Autodesk Inventor part; units mm, degrees
ref_plane "Work Plane1" through (0, 0, 10) normal (0, 0, 1) x (1, 0, 0)
ref_plane "YZ Plane" through (0, 0, 0) normal (1, 0, 0) x (0, 1, 0)
ref_plane "XZ Plane" through (0, 0, 0) normal (0, 1, 0) x (-1, 0, 0)
ref_plane "Work Plane1" through (0, 0, 10) normal (0, 0, 1) x (1, 0, 0)
sketch "Sketch1" plane through (0, 0, 10) normal (0, 0, 1) x (1, 0, 0)
  line L0 (-4.0299, -0.3538) -> (-2.2322, 1.4439) construction
  arc A0 (-1.4439, 2.2322) -> (-2.2322, 1.4439) centre (-0.9299, 0.9299) ccw construction
  line L1 (-1.4439, 2.2322) -> (0.3538, 4.0299) construction
  line L2 (-37.8299, 42.8299) -> (-37.8299, 37.8299) construction
  line L3 (-37.8299, 37.8299) -> (-42.9208, 37.8299) construction
  line L4 (-37.8299, 42.2137) -> (-37.8299, 45.8299) construction
  line L5 (-37.8299, 45.8299) -> (-4.0299, 45.8299) construction
  line L6 (-4.0299, 45.8299) -> (-4.0299, 42.2137) construction
  line L7 (-4.0299, 4.0299) -> (0.3538, 4.0299)
  circle A1 centre (-20.9299, 20.9299) radius 17.5
  line L8 (-20.9299, 58.9723) -> (17.1124, 20.9299) construction
  line L9 (17.1124, 20.9299) -> (-20.9299, -17.1124) construction
  line L10 (-20.9299, -17.1124) -> (-58.9723, 20.9299) construction
  line L11 (-58.9723, 20.9299) -> (-20.9299, 58.9723) construction
  line L12 (-20.9299, 58.9723) -> (-20.9299, -17.1124) construction
  line L13 (17.1124, 20.9299) -> (-58.9723, 20.9299) construction
  line L14 (-20.9299, 58.9723) -> (32.8701, 58.9723) construction
  line L15 (-43.4299, 43.4299) -> (1.5701, 43.4299) construction
  line L16 (1.5701, 43.4299) -> (1.5701, -1.5701) construction
  line L17 (1.5701, -1.5701) -> (-43.4299, -1.5701) construction
  line L18 (-43.4299, -1.5701) -> (-43.4299, 43.4299) construction
  line L19 (-43.4299, 43.4299) -> (1.5701, -1.5701) construction
  line L20 (1.5701, 43.4299) -> (-43.4299, -1.5701) construction
  line L21 (-43.4299, 5.3876) -> (-43.4299, 36.4723)
  line L22 (-43.4299, 36.4723) -> (-36.4723, 43.4299)
  line L23 (-36.4723, 43.4299) -> (-5.3876, 43.4299)
  line L24 (-5.3876, 43.4299) -> (1.5701, 36.4723)
  line L25 (1.5701, 36.4723) -> (1.5701, 5.3876)
  line L26 (1.5701, 5.3876) -> (-5.3876, -1.5701)
  line L27 (-5.3876, -1.5701) -> (-36.4723, -1.5701)
  line L28 (-36.4723, -1.5701) -> (-43.4299, 5.3876)
  line L29 (-4.0299, 42.2137) -> (-37.8299, 42.2137)
  line L30 (-4.0299, -0.3538) -> (-4.0299, 4.0299)
  circle A2 centre (-20.9299, 20.9299) radius 1.5
  line L31 (-10.9299, 10.9299) -> (-30.9299, 10.9299) construction
  line L32 (-30.9299, 10.9299) -> (-30.9299, 30.9299) construction
  line L33 (-30.9299, 30.9299) -> (-10.9299, 30.9299) construction
  line L34 (-10.9299, 30.9299) -> (-10.9299, 10.9299) construction
  line L35 (-10.9299, 10.9299) -> (-30.9299, 30.9299) construction
  line L36 (-30.9299, 10.9299) -> (-10.9299, 30.9299) construction
  circle A3 centre (-30.9299, 30.9299) radius 1.4
  circle A4 centre (-30.9299, 10.9299) radius 1.4
  circle A5 centre (-10.9299, 10.9299) radius 1.4
  line L37 (-45.8299, 37.8299) -> (-42.0723, 37.8299) construction
  line L38 (-42.1723, 37.7299) -> (-45.8299, 37.7299)
  line L39 (-45.8299, 37.7299) -> (-45.8299, 4.1299)
  line L40 (-45.8299, 4.1299) -> (-42.1723, 4.1299)
  line L41 (-42.1723, 4.1299) -> (-42.1723, 37.7299)
  line L42 (-45.8299, 4.0299) -> (-42.0723, 4.0299) construction
  line L43 (-45.8299, 37.8299) -> (-42.0723, 37.8299)
  line L44 (-37.7299, 45.8299) -> (-4.1299, 45.8299)
  line L45 (-4.1299, 45.8299) -> (-4.1299, 42.1723)
  line L46 (-4.1299, 42.1723) -> (-37.7299, 42.1723)
  line L47 (-37.7299, 42.1723) -> (-37.7299, 45.8299)
  line L48 (0.4701, 37.8299) -> (0.4701, 4.0299) construction
  line L49 (0.4701, 4.0299) -> (3.9701, 4.0299) construction
  line L50 (3.9701, 37.8299) -> (3.9701, 4.0299) construction
  line L51 (0.4701, 37.8299) -> (3.9701, 37.8299) construction
  line L52 (-45.8299, -3.9701) -> (-4.0299, -3.9701) construction
  line L53 (0.3124, 37.7299) -> (3.9701, 37.7299)
  line L54 (3.9701, 37.7299) -> (3.9701, 4.1299)
  line L55 (3.9701, 4.1299) -> (0.3124, 4.1299)
  line L56 (0.3124, 4.1299) -> (0.3124, 37.7299)
  line L57 (-4.1713, -0.3538) -> (-37.7299, -0.3538)
  line L58 (-37.7299, -0.3538) -> (-37.7299, -3.9701)
  line L59 (-37.7299, -3.9701) -> (-4.1713, -3.9701)
  line L60 (-4.1713, -3.9701) -> (-4.1713, -0.3538)
  point P0 (-37.8299, 4.0299)
  dimension "d18" = 53.8
  dimension "d19" = 45
  dimension "d20" = 53.8
  dimension "d21" = 45
  dimension "d22" = 45
  dimension "d30" = 20
  dimension "d31" = 20
  dimension "d32" = 2.8
  dimension "d33" = 2.8
  dimension "d34" = 2.8
  dimension "d35" = 3
  dimension "d36" = 0.1
  dimension "d37" = 0.1
  dimension "d38" = 0.1
  dimension "d39" = 0.1
extrude "Extrusion1" add sketch "Sketch1" along normal blind 11 contours L30 L26 L57 L28 L41 L22 L46 L24 L56 L7 | L7 L26 L30 | L56 L24 L25 L26 | L26 L25 L24 L53 L54 L55 | L60 L59 L58 L57 L28 L27 L26 | L26 L27 L28 L57 | L46 L22 L29 L24 | L24 L29 L45 | L40 L39 L38 L22 L21 L28 | L28 L21 L22 L41 | L29 L22 L23 L24 | L24 L23 L22 L29 L47 L44 L45 | L47 L29 L22 | A1 | A2 | A3 | A4 | A5
sketch "Skizze4" plane through (0, 0, 21) normal (0, 0, 1) x (1, 0, 0)
  line L0 (-37.7299, 42.1723) -> (-42.1723, 37.7299)
  line L1 (-42.1723, 37.7299) -> (-45.8299, 37.7299)
  line L2 (-45.8299, 37.7299) -> (-45.8299, 4.1299) construction
  line L3 (-45.8299, 4.1299) -> (-42.1723, 4.1299)
  line L4 (-42.1723, 4.1299) -> (-37.6885, -0.3538)
  line L5 (-37.6885, -0.3538) -> (-37.7299, -0.3538)
  line L6 (-37.7299, -0.3538) -> (-37.7299, -3.9701)
  line L7 (-37.7299, -3.9701) -> (-4.1713, -3.9701) construction
  line L8 (-4.1713, -3.9701) -> (-4.1713, -0.3538)
  line L9 (-4.1713, -0.3538) -> (0.3124, 4.1299)
  line L10 (0.3124, 4.1299) -> (3.9701, 4.1299)
  line L11 (3.9701, 4.1299) -> (3.9701, 37.7299) construction
  line L12 (3.9701, 37.7299) -> (0.3124, 37.7299)
  line L13 (0.3124, 37.7299) -> (-4.1299, 42.1723)
  line L14 (-4.1299, 42.1723) -> (-4.1299, 45.8299)
  line L15 (-4.1299, 45.8299) -> (-37.7299, 45.8299) construction
  line L16 (-37.7299, 45.8299) -> (-37.7299, 42.1723)
  line L17 (-37.9299, 46.0299) -> (-3.9299, 46.0299) construction
  line L18 (-3.9299, 46.0299) -> (-3.9299, 42.2551)
  line L19 (-3.9299, 42.2551) -> (0.3953, 37.9299)
  line L20 (0.3953, 37.9299) -> (4.1701, 37.9299)
  line L21 (4.1701, 37.9299) -> (4.1701, 3.9299) construction
  line L22 (4.1701, 3.9299) -> (0.3953, 3.9299)
  line L23 (0.3953, 3.9299) -> (-3.9713, -0.4367)
  line L24 (-3.9713, -0.4367) -> (-3.9713, -4.1701)
  line L25 (-3.9713, -4.1701) -> (-37.9299, -4.1701) construction
  line L26 (-37.9299, -4.1701) -> (-37.9299, -0.3953)
  line L27 (-37.9299, -0.3953) -> (-42.2551, 3.9299)
  line L28 (-42.2551, 3.9299) -> (-46.0299, 3.9299)
  line L29 (-46.0299, 3.9299) -> (-46.0299, 37.9299) construction
  line L30 (-46.0299, 37.9299) -> (-42.2551, 37.9299)
  line L31 (-42.2551, 37.9299) -> (-37.9299, 42.2551)
  line L32 (-37.9299, 42.2551) -> (-37.9299, 46.0299)
  line L33 (-45.8299, 37.7299) -> (-45.8299, 37.9299)
  line L34 (-4.1299, 45.8299) -> (-37.7299, 45.8299)
  line L35 (-37.7299, 45.8299) -> (-37.9299, 45.8299)
  line L36 (-4.1299, 45.8299) -> (-3.9299, 45.8299)
  line L37 (3.9701, 37.7299) -> (3.9701, 37.9299)
  line L38 (3.9701, 4.1299) -> (3.9701, 37.7299)
  line L39 (3.9701, 4.1299) -> (3.9701, 3.9299)
  line L40 (-4.1713, -3.9701) -> (-3.9713, -3.9701)
  line L41 (-37.7299, -3.9701) -> (-37.9299, -3.9701)
  line L42 (-45.8299, 4.1299) -> (-45.8299, 3.9299)
  point P0 (0, 0)
  dimension "d40" = 0.2
extrude "IM_offset" add sketch "Skizze4" against normal up to surface (11 mm away)
ref_plane "Arbeitsebene5" through (-20.9299, 3.9299, 10) normal (1, 0, 0) x (0, 0, -1)
ref_plane "Arbeitsebene6" through (-37.9299, 20.9299, 10) normal (0, 1, 0) x (1, 0, 0)
sketch "Skizze25" plane through (0, 0, 21) normal (0, 0, 1) x (1, 0, 0)
  arc A0 (-35.9433, 11.4849) -> (-11.4049, 36.0233) centre (-20.9299, 21.0099) ccw
  circle A1 centre (-20.9299, 21.0099) radius 17.78
  circle A2 centre (-20.9299, 21.0099) radius 13
  point P0 (0, 0)
  point P1 (-11.4049, 36.0233)
  dimension "d152" = 26
extrude "Extrusion21" cut sketch "Skizze25" against normal blind 12 contours A2
sketch "Skizze26" plane through (0, 0, 21) normal (0, 0, 1) x (1, 0, 0)
  line L0 (-43.7899, 28.1537) -> (-43.7899, 13.8662)
  arc A0 (-43.7899, 13.8662) -> (-41.4087, 11.4849) centre (-41.4087, 13.8662) ccw
  line L1 (-41.4087, 11.4849) -> (-35.9433, 11.4849)
  arc A1 (-35.9433, 11.4849) -> (-11.4049, 36.0233) centre (-20.9299, 21.0099) ccw
  line L2 (-11.4049, 36.0233) -> (-11.4049, 41.4887)
  arc A2 (-11.4049, 41.4887) -> (-13.7862, 43.8699) centre (-13.7862, 41.4887) ccw
  line L3 (-13.7862, 43.8699) -> (-28.0737, 43.8699)
  arc A3 (-28.0737, 43.8699) -> (-30.4549, 41.4887) centre (-28.0737, 41.4887) ccw
  line L4 (-30.4549, 41.4887) -> (-30.4549, 36.0233)
  arc A4 (-30.4549, 36.0233) -> (-35.9433, 30.5349) centre (-20.9299, 21.0099) ccw
  line L5 (-35.9433, 30.5349) -> (-41.4087, 30.5349)
  arc A5 (-41.4087, 30.5349) -> (-43.7899, 28.1537) centre (-41.4087, 28.1537) ccw
  circle A6 centre (-20.9299, 21.0099) radius 13.2911
  point P0 (0, 0)
extrude "Extrusion22" cut sketch "Skizze26" against normal blind 9.2 contours A5 L5 A4 L4 A3 L3 A2 L2 A1 L1 A0 L0 | A6
sketch "Skizze27" plane through (-37.9299, -3.9701, 10) normal (0, -1, 0) x (1, 0, 0)
  line L0 (33.9586, 0) -> (0, 0)
  line L1 (33.9586, 11) -> (33.9586, 0)
  line L2 (33.9586, 11) -> (0, 11)
  line L3 (0, 11) -> (0, 0)
  circle A0 centre (16.9793, 6) radius 2.85
  point P0 (37.9299, -10)
  dimension "d155" = 5.7
hole "Bohrung1" at (-20.9506, -3.9701, 16) direction (0, 1, 0) diameter 4.5 depth 30 tip angle 118 counterbore diameter 5.7 counterbore depth 5.8
sketch "Skizze28" plane through (0, 0, 21) normal (0, 0, 1) x (1, 0, 0)
  line L0 (-35.9433, 11.4849) -> (-41.4087, 11.4849)
  arc A0 (-43.7899, 13.8662) -> (-41.4087, 11.4849) centre (-41.4087, 13.8662) ccw
  line L1 (-43.7899, 13.8662) -> (-43.7899, 28.1537)
  arc A1 (-41.4087, 30.5349) -> (-43.7899, 28.1537) centre (-41.4087, 28.1537) ccw
  line L2 (-41.4087, 30.5349) -> (-35.9433, 30.5349)
  arc A2 (-30.4549, 36.0233) -> (-35.9433, 30.5349) centre (-20.9299, 21.0099) ccw
  line L3 (-30.4549, 36.0233) -> (-30.4549, 41.4887)
  arc A3 (-28.0737, 43.8699) -> (-30.4549, 41.4887) centre (-28.0737, 41.4887) ccw
  line L4 (-28.0737, 43.8699) -> (-13.7862, 43.8699)
  arc A4 (-11.4049, 41.4887) -> (-13.7862, 43.8699) centre (-13.7862, 41.4887) ccw
  line L5 (-11.4049, 41.4887) -> (-11.4049, 36.0233)
  arc A5 (-35.9433, 11.4849) -> (-11.4049, 36.0233) centre (-20.9299, 21.0099) ccw
  line L6 (3.9701, 3.9299) -> (3.9701, 37.9299)
  line L7 (3.9701, 37.9299) -> (0.3953, 37.9299)
  line L8 (0.3953, 37.9299) -> (-3.9299, 42.2551)
  line L9 (-3.9299, 42.2551) -> (-3.9299, 45.8299)
  line L10 (-3.9299, 45.8299) -> (-37.9299, 45.8299)
  line L11 (-37.9299, 45.8299) -> (-37.9299, 42.2551)
  line L12 (-37.9299, 42.2551) -> (-42.2551, 37.9299)
  line L13 (-42.2551, 37.9299) -> (-45.8299, 37.9299)
  line L14 (-45.8299, 37.9299) -> (-45.8299, 3.9299)
  line L15 (-42.2551, 3.9299) -> (-45.8299, 3.9299)
  line L16 (-37.9299, -0.3953) -> (-42.2551, 3.9299)
  line L17 (-37.9299, -3.9701) -> (-37.9299, -0.3953)
  line L18 (-3.9713, -3.9701) -> (-37.9299, -3.9701)
  line L19 (-3.9713, -3.9701) -> (-3.9713, -0.4367)
  line L20 (-3.9713, -0.4367) -> (0.3953, 3.9299)
  line L21 (0.3953, 3.9299) -> (3.9701, 3.9299)
  circle A6 centre (-1.2449, 9.5799) radius 2.0828
  circle A7 centre (-1.2449, 32.4399) radius 2.0828
  circle A8 centre (-40.6149, 32.4399) radius 2.0828
  circle A9 centre (-40.6149, 9.5799) radius 2.0828
  point P0 (0, 0)
hole "Bohrung2" at (-40.6149, 9.5799, 21) at (-40.6149, 32.4399, 21) at (-1.2449, 32.4399, 21) at (-1.2449, 9.5799, 21) direction (0, 0, -1) diameter 2.8 depth 30 tip angle 118
sketch "Skizze29" plane through (-28.0737, 43.8699, 21) normal (0, -1, 0) x (1, 0, 0)
  circle A0 centre (7.123, -5) radius 2.85
  circle A1 centre (7.123, -5) radius 4.25
  point P0 (28.0737, -21)
  dimension "d173" = 8.5
extrude "Extrusion23" cut sketch "Skizze29" against normal blind 1 contours A0 | A1
pattern_circular "Runde Anordnung1" count 2 over 90 about axis through (-20.9299, 21.0099, 21) along (0, 0, 1) of "Bohrung1", "Extrusion23"
properties part number "20_Cube_Insert_Filter_25mm"
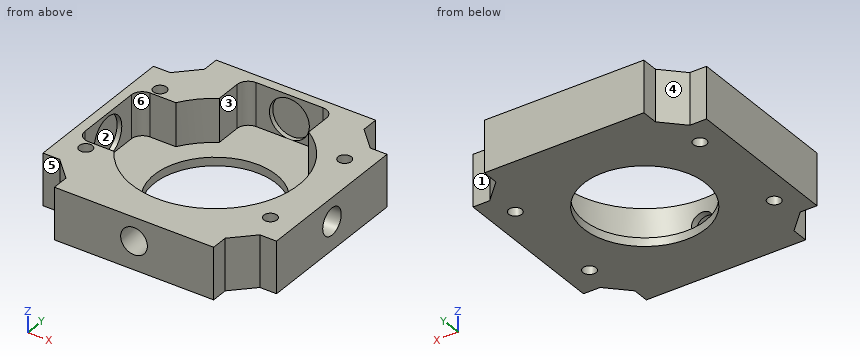
Geometry: final body of the model. Coordinates: model frame, mm. Face numbers are marked on the shaded views. A direction names the side the tool comes from. Round coordinates to 2 decimals unless told otherwise and drop trailing zeros. Order: outer loops, then holes, each group sorted by start corner. A loop starts at its lowest first (then second) coordinate and runs counter-clockwise, first axis right, second up. Notation, with made-up numbers: (-18.5, -10) - (17.5, -10) arc R22 ccw to (17.5, 12) - close; hole circle Ø7 at (60, 2). An arc over 180 degrees is marked (long way). Use CSV: the item, a comma, the result in double quotes. Start each with the question number.
Q1. First-contact query: pin 1 (1.1 mm diameter, centred on x = -44.5, z = 13.5, fed in from -Y); pin 2 (1.6 mm diameter, centred on x = -39, z = 16.5, fed in from -Y); pin 3 (1.1 mm diameter, centred on x = -45, z = 13, fed in from +Y). Flat tips, straight axial feed; report the tip coordinate or a pass-through.
Q2. Access query for the marked faces 1, 2 and 3. Directions: +Z, -Z, +X, -X, +Y, -Y. A direction counts if a zero-diameter tool reaches every point of the face in a straight line with its end or side. Return the directions, or none.
Q3. Material intervals for line 1 along Y through (x, z) = (-16, 13.5); line 2 along X through (y, z) = (9, 19); line 3 along X through (y, z) = (44.35, 16), sorted ascending. Write a range as from..to.
Q4. Section query A-A (y = 27.5). Return loops of the section in (x, z), and give its area (3 significant figures).
Q5. Section query B-B (x = -32.5). Return loops of the section in (y, z), and give its area (3 significant figures).
Q6. Mould query, pull axis Y, two halves, no side actions, for the marked faces 4, 5 and 6. Classes: +Y half, -Y half, draft (parallel to the pull), parting line (faces both ways), or undercut.
Q7. Section query C-C (x = -19.5). Return loops of the section in (y, z), and give its area (3 significant figures).
Q8. Section query D-D (z = 17.5). State how many separate pieces and enclosed holes the cut face has, and give its area (3 significant figures).
Result set:
1,pin 1,"stops at y = 3.93"
1,pin 2,"stops at y = -0.13"
1,pin 3,"stops at y = 37.93"
2,face 1,"+Z, -Z, +X, +Y"
2,face 2,"none"
2,face 3,"+Z"
3,line 1,"y = -3.97..3.93, 43.87..45.83"
3,line 2,"x = -45.83..-41.89, -39.34..-34.04, -7.82..-2.52, 0.03..3.97"
3,line 3,"x = -37.93..-25.2, -16.7..-3.93"
4,outline,"(-45.83, 10) - (-32.19, 10) - (-32.19, 11.8) - (-43.79, 11.8) - (-43.79, 21) - (-45.83, 21) - close; (-9.67, 10) - (3.97, 10) - (3.97, 21) - (-4.38, 21) - (-4.38, 11.8) - (-9.67, 11.8) - close"
4,area,"145 mm2"
5,outline,"(-3.97, 10) - (15.08, 10) - (15.08, 11.8) - (7.51, 11.8) - (7.51, 21) - (-3.97, 21) - close; (26.94, 10) - (45.83, 10) - (45.83, 21) - (34.51, 21) - (34.51, 11.8) - (26.94, 11.8) - close"
5,area,"278 mm2"
6,face 4,"+Y half"
6,face 5,"-Y half"
6,face 6,"undercut"
7,outline,"(-3.97, 10) - (8.09, 10) - (8.09, 11.8) - (3.29, 11.8) - (3.29, 14.28) - (1.83, 14.28) - (1.83, 13.55) - (-3.97, 13.55) - close; (-3.97, 18.45) - (1.83, 18.45) - (1.83, 17.72) - (3.29, 17.72) - (3.29, 21) - (-3.97, 21) - close; (33.93, 10) - (45.83, 10) - (45.83, 21) - (43.87, 21) - (43.87, 19.99) - (44.87, 19.99) - (44.87, 12.01) - (43.87, 12.01) - (43.87, 11.8) - (33.93, 11.8) - close"
7,area,"86.5 mm2"
8,separate pieces,"2"
8,enclosed holes,"4"
8,area,"946 mm2"
